```python
from build123d import *
from build123d.topology import SkipClean

# Parameters (mm, degrees)
SKETCH2_R           = 4.7625
BOSS_EXTRUDE1_DEPTH = 3.81
SKETCH3_R           = 3.175
BOSS_EXTRUDE2_DEPTH = 25.4
THREAD2_PITCH       = 1.27
THREAD2_HEIGHT      = 6.35
THREAD2_RADIUS      = 3.175
THREAD2_START_ANGLE = 90


with BuildPart() as part:
    # Sketch2 → Boss-Extrude1 (new body)
    with BuildSketch(Plane(origin=(0, 0, 0), x_dir=(1, 0, 0), z_dir=(0, 1, 0))):
        with Locations(Location((0, 0, 0), (0, 0, 90))):
            Circle(SKETCH2_R)
    extrude(amount=BOSS_EXTRUDE1_DEPTH)

    # Sketch3 → Boss-Extrude2 (add)
    with BuildSketch(Plane(origin=(0, 3.81, 0), x_dir=(1, 0, 0), z_dir=(0, 1, 0))):
        with Locations(Location((0, 0, 0), (0, 0, 270))):
            Circle(SKETCH3_R)
    extrude(amount=BOSS_EXTRUDE2_DEPTH)

    # Thread2: sweep along a helix
    with SkipClean():  # the faces are left unmerged after this step: merging them gives an invalid solid
        with BuildLine() as thread2_path:
            add(Helix(THREAD2_PITCH, THREAD2_HEIGHT, THREAD2_RADIUS, center=(0, 3.81, 0), direction=(0, 1, 0), mode=Mode.PRIVATE).rotate(Axis((0, 3.81, 0), (0, 1, 0)), THREAD2_START_ANGLE))
        # Thread Profile2 → Thread2 (sweep)
        with BuildSketch(Plane(origin=(3.175, 3.81, 0), x_dir=(1, 0, 0), z_dir=(0, 0, 1))):
            Polygon((0, 0), (0.687407661, 0.396874998), (0.687407661, 0.555624998), (0, 0.952499997), align=None)
        sweep(path=thread2_path.line, is_frenet=True)


solid = part.part
```
The listing builds one solid part. Answer for the finished solid, in the listing's coordinates (mm). Coordinates: 2 decimals unless noted, no trailing zeros. Loops run counter-clockwise (first coordinate to the right, second up) from the corner with the lowest first, then second, coordinate; pieces in that order, holes last. Notation, with made-up numbers: M 30,-25 L 68,-25 A30 cw 68,14 Z; hole C 86.5,11 d1. An arc over 180 degrees is marked long. Answer as a JSON object with one key per item and string values. Group by question number.
Item 1: Section B-B (y = 3.5) is taken. Write down the section's boundary in (x, z) (1 decimal).
Item 2: Section A-A (y = 21.25) is taken. Write down the section's boundary in (x, z) (3 decimals).
Item 3: Consider L1, parallel to Y at x = -3, z = -2.25; L2, parallel to Y at x = -3.75, z = 1.75; L3, parallel to X at y = 16, z = 1. Determine where each line is inside the solid, lowest interval first.
Item 4: Each of these flat-tipped pins is pushed along its axis until it touches: P1, Ø5, axis at y = 8, z = 3, coming from the +X side; P2, Ø4, axis at x = 0, y = 10.5, coming from the +Z side; P3, Ø1, axis at x = 2, z = 1.5, coming from the -Y side; P4, Ø1, axis at x = -3, y = 21, coming from the -Z side. Where does it stop, or does it pass through?
Solved:
{
 "1": {"outline": "C 0,0 d9.5"},
 "2": {"outline": "C 0,0 d6.35"},
 "3": {"L1": "y = 0 to 3.81, 4.65 to 4.94, 5.92 to 6.21, 7.19 to 7.48, 8.46 to 8.75, 9.73 to 10.02", "L2": "y = 0 to 3.81", "L3": "x = -3.01 to 3.01"},
 "4": {"P1": "stops at x = 3.83", "P2": "stops at z = 3.86", "P3": "stops at y = 0", "P4": "stops at z = -1.96"}
}
